Build history of the part. All positions in model axes, mm. Give positions to 0.01 mm unless a question says otherwise; leave off trailing zeros. Loops run counter-clockwise (first coordinate to the right, second up) from the corner with the lowest first, then second, coordinate; pieces in that order, holes last. Notation, with made-up numbers: (26, -3) - (56, -3) arc R20 ccw to (56, 8) - close; hole circle Ø3 at (88, -23.75). An arc over 180 degrees is marked (long way). Return JSON: item names as keys, results as strings. Group by question number.
1) Slice it at B-B (y = -76.5). List the corners of the cut face in (x, z).
2) Slice it at C-C (x = 78). List the corners of the cut face in (y, z), and give its area (3 significant figures).
3) Slice it at A-A (x = 45.5). List the corners of the cut face in (y, z).
4) Mould opens along X. For faces 1 (the face through (93, -39, 1)), 2 (the face through (-2, -40, 1)), 3 (the face through (5, -41, 1)), 4 (the face through (46, -80.5, 1)) say: released by +X, released by -X, zero draft, split by the parting line, or undercut.
5) Drill centre lines: probe 1 along X at (y, z) = (-76.5, 0.8); probe 2 along Y at (x, z) = (45.5, 1.35); probe 3 along Y at (x, z) = (13, 1.1). Where is each one in solid material? Low to high. Write a range as from..to.
Autodesk Inventor part; units mm, degrees
ref_plane "YZ Plane" through (0, 0, 0) normal (1, 0, 0) x (0, 1, 0)
ref_plane "XZ Plane" through (0, 0, 0) normal (0, 1, 0) x (-1, 0, 0)
ref_plane "XY Plane" through (0, 0, 0) normal (0, 0, 1) x (1, 0, 0)
ref_plane "Work Plane1" through (0, 0, 0) normal (0, 0, 1) x (1, 0, 0)
sketch "Sketch1" plane through (0, 0, 0) normal (0, 0, 1) x (1, 0, 0)
  line L0 (93, -80.5) -> (83, -80.5)
  line L1 (93, 2) -> (93, -80.5)
  line L2 (-2, -80.5) -> (-2, 2)
  line L3 (0, 2) -> (-2, 2)
  circle A0 centre (45.5, -4) radius 0.75
  circle A1 centre (81, -4) radius 0.75
  circle A2 centre (10, -4) radius 0.75
  circle A3 centre (4, -40.25) radius 0.75
  circle A4 centre (4, -70.5) radius 0.75
  circle A5 centre (87, -40.25) radius 0.75
  circle A6 centre (81, -76.5) radius 1.25
  circle A7 centre (45.5, -76.5) radius 1.25
  circle A8 centre (10, -76.5) radius 1.25
  line L4 (93, -80.5) -> (-2, -80.5)
  line L5 (-2, -80.5) -> (-2, 2)
  line L6 (-2, 2) -> (93, 2)
  line L7 (93, 2) -> (93, -80.5)
  point P0 (0, 0)
  point P1 (87.75, -75.5)
extrude "Extrusion1" add sketch "Sketch1" along normal blind 2
sketch "Sketch2" plane through (0, 0, 2) normal (0, 0, 1) x (1, 0, 0)
  circle A0 centre (4, -70.5) radius 0.75
  circle A1 centre (4, -70.5) radius 1.25
  circle A2 centre (4, -40.25) radius 0.75
  circle A3 centre (4, -40.25) radius 1.25
  circle A4 centre (10, -4) radius 0.75
  circle A5 centre (10, -4) radius 1.25
  circle A6 centre (45.5, -4) radius 0.75
  circle A7 centre (45.5, -4) radius 1.25
  circle A8 centre (81, -4) radius 0.75
  circle A9 centre (81, -4) radius 1.25
  circle A10 centre (87, -40.25) radius 0.75
  circle A11 centre (87, -40.25) radius 1.25
  point P0 (0, 0)
  dimension "d2" = 2.5
  dimension "d3" = 2.5
  dimension "d4" = 2.5
  dimension "d5" = 2.5
  dimension "d6" = 2.5
  dimension "d7" = 2.5
extrude "Extrusion2" cut sketch "Sketch2" against normal blind 2
sketch "Sketch3" plane through (0, 0, 2) normal (0, 0, 1) x (1, 0, 0)
  circle A0 centre (4, -70.5) radius 1.25
  circle A1 centre (4, -70.5) radius 1.25
  point P0 (0, 0)
extrude "Extrusion3" add sketch "Sketch3" against normal blind 2
sketch "Sketch4" plane through (0, 0, 2) normal (0, 0, 1) x (1, 0, 0)
  line L0 (8.2244, -73.6994) -> (84.6233, -73.6994)
  line L1 (84.6233, -73.6994) -> (84.6233, -78.8307)
  line L2 (84.6233, -78.8307) -> (8.2244, -78.8307)
  line L3 (8.2244, -78.8307) -> (8.2244, -73.6994)
  point P0 (0, 0)
extrude "Extrusion4" add sketch "Sketch4" against normal blind 2
sketch "Sketch5" plane through (0, 0, 2) normal (0, 0, 1) x (1, 0, 0)
  line L0 (3.25, -80.5) -> (3.25, -75.5)
  line L1 (83, -80.5) -> (83, -65.5)
  circle A0 centre (45.5, -76.5) radius 1.25
  line L2 (83, -72.5) -> (83, -80.5)
  circle A1 centre (78, -76.5) radius 1.25
  line L3 (8, -80.5) -> (8, -65.5)
  line L4 (8, -72.5) -> (8, -80.5)
  circle A2 centre (13, -76.5) radius 1.25
  point P0 (0, 0)
  dimension "d21" = 2.5
  dimension "d25" = 2.5
extrude "Extrusion5" cut sketch "Sketch5" against normal blind 2
properties part number "UP" material "Nylon 6/6"
Results:
{
 "1": {"outline": "(-2, 0) - (11.75, 0) - (11.75, 2) - (-2, 2) - close; (14.25, 0) - (44.25, 0) - (44.25, 2) - (14.25, 2) - close; (46.75, 0) - (76.75, 0) - (76.75, 2) - (46.75, 2) - close; (79.25, 0) - (93, 0) - (93, 2) - (79.25, 2) - close"},
 "2": {"outline": "(-80.5, 0) - (-77.75, 0) - (-77.75, 2) - (-80.5, 2) - close; (-75.25, 0) - (2, 0) - (2, 2) - (-75.25, 2) - close", "area": "160 mm2"},
 "3": {"outline": "(-80.5, 0) - (-77.75, 0) - (-77.75, 2) - (-80.5, 2) - close; (-75.25, 0) - (-5.25, 0) - (-5.25, 2) - (-75.25, 2) - close; (-2.75, 0) - (2, 0) - (2, 2) - (-2.75, 2) - close"},
 "4": {"face 1": "released by +X", "face 2": "released by -X", "face 3": "undercut", "face 4": "zero draft"},
 "5": {"probe 1": "-2..11.75, 14.25..44.25, 46.75..76.75, 79.25..93", "probe 2": "-80.5..-77.75, -75.25..-5.25, -2.75..2", "probe 3": "-80.5..-77.75, -75.25..2"}
}
